Here's the drawing with two shaded views (mm, measured from the low corner). I have some questions. A direction names the side the tool comes from. Coordinates: 2 decimals unless noted, no trailing zeros. Order: outer loops, then holes, each group sorted by start corner. A loop starts at its lowest first (then second) coordinate and runs counter-clockwise, first axis right, second up. Notation, with made-up numbers: (12.5, 37.25) - (65.5, 37.25) arc R31 ccw to (65.5, 62.25) - close; hole circle Ø8 at (5.5, -3). An arc over 180 degrees is marked (long way). Answer as CSV lines item,"result". Start each with the question number.
1. I need wall thicknesses on probe 1 along Z at (x, y) = (7, 3.3) (1 decimal); probe 2 along Z at (x, y) = (6, 2.8); probe 3 along X at (y, z) = (2.25, 7.5) (1 decimal). Which ranges of each line are inside material? Lowest first, please.
2. Thinking about a two-plate mould opening in X: for the marked faces 5, 6, 7 and 8, which applies, released by +X, released by -X, zero draft, split by the parting line, or undercut?
3. For the marked faces 1, 2, 3 and 4, which set-ups out of +Z, -Z, +X, -X, +Y, -Y let a thin tool reach every point of the face, with its end or its side?
4. I want a section at C-C, the plane x = 5.25. List the corners of the cut face in (y, z) for me (1 decimal).
5. I want a section at D-D, the plane x = 9.5. List the corners of the cut face in (y, z) for me (1 decimal).
6. I want a section at B-B, the plane y = 1.85. List the corners of the cut face in (x, z) for me (1 decimal).
7. For pin 1 (1 mm diameter, centred on x = 5.5, z = 6, fed in from -Y); pin 2 (2 mm diameter, centred on y = 1, z = 6.5, fed in from -X); pin 3 (1.5 mm diameter, centred on x = 5.5, y = 3, fed in from +Z); pin 4 (1.5 mm diameter, centred on y = 0.5, z = 5, fed in from +X), each with a flat end and sliding along its axis, tell me the tip position at first contact or that it passes through.
8. I want a section at A-A, the plane z = 1. List the corners of the cut face in (x, y) for me (1 decimal).
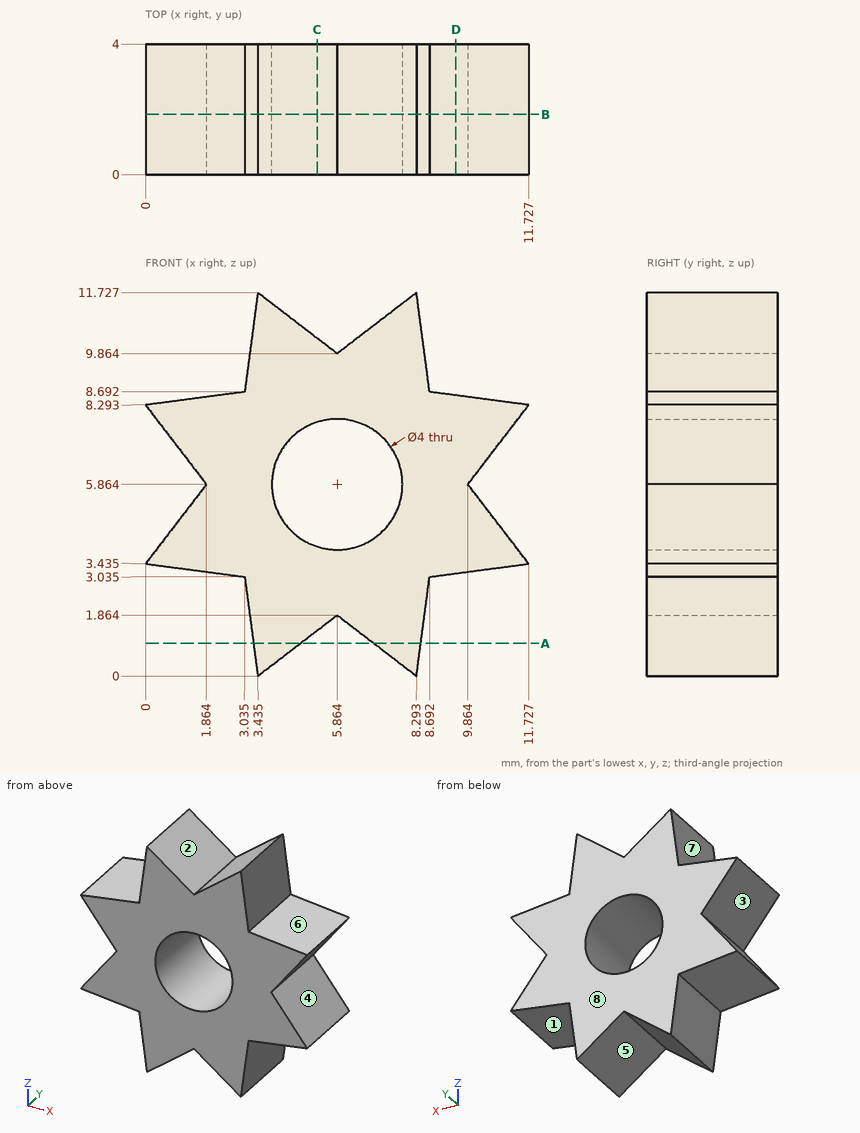
Solved:
1,probe 1,"z = 1 to 4.2, 7.5 to 10.7"
1,probe 2,"z = 1.76 to 3.87, 7.86 to 9.97"
1,probe 3,"x = 0.6 to 4.7, 7 to 11.1"
2,face 5,"undercut"
2,face 6,"released by +X"
2,face 7,"released by -X"
2,face 8,"zero draft"
3,face 1,"-Z, +X, +Y, -Y"
3,face 2,"+Z, +Y, -Y"
3,face 3,"-X, +Y, -Y"
3,face 4,"+X, +Y, -Y"
4,outline,"(0, 1.4) - (4, 1.4) - (4, 4) - (0, 4) - close; (0, 7.8) - (4, 7.8) - (4, 10.3) - (0, 10.3) - close"
5,outline,"(0, 3.1) - (4, 3.1) - (4, 8.6) - (0, 8.6) - close"
6,outline,"(0, 3.4) - (3, 3) - (3.4, 0) - (5.9, 1.9) - (8.3, 0) - (8.7, 3) - (11.7, 3.4) - (9.9, 5.9) - (11.7, 8.3) - (8.7, 8.7) - (8.3, 11.7) - (5.9, 9.9) - (3.4, 11.7) - (3, 8.7) - (0, 8.3) - (1.9, 5.9) - close; hole circle Ø4 at (5.9, 5.9)"
7,pin 1,"passes through"
7,pin 2,"stops at x = 0.61"
7,pin 3,"stops at z = 10.72"
7,pin 4,"stops at x = 11.1"
8,outline,"(3.3, 0) - (4.7, 0) - (4.7, 4) - (3.3, 4) - close; (7, 0) - (8.4, 0) - (8.4, 4) - (7, 4) - close"
